Answer from the drawing. Dimensions are ordinates in mm from the lowest x, y and z of the part. A direction names the side the tool comes from. Coordinates: 2 decimals unless noted, no trailing zeros. Order: outer loops, then holes, each group sorted by start corner. A loop starts at its lowest first (then second) coordinate and runs counter-clockwise, first axis right, second up. Notation, with made-up numbers: M 42.5,7.25 L 48.5,7.25 A22 cw 48.5,24.25 Z; hole C 53.5,17.25 d7. An arc over 180 degrees is marked long. One line per question, with ' | ' between items. Start each with the question number.
1) Find section A-A, the plane z = 3. Write down the section's boundary in (x, y).
2) Find section B-B, the plane y = 3. Write down the section's boundary in (x, z).
3) Given P1, Ø0.9, axis at x = 4, z = 3, coming from the +Y side; P2, Ø1, axis at y = 3, z = 5, coming from the +X side; P3, Ø2, axis at x = 1.5, y = 21.5, coming from the +Z side, each flat-ended and moving along its own axis, determine where each tip first touches the part or whether it passes through.
4) Consider probe 1 along Y at (x, z) = (4.95, 3); probe 2 along Z at (x, y) = (4, 15.75); probe 3 along Z at (x, y) = (2.9, 16). Determine where each line is inside the solid, lowest interval first.
5) A tool of negligible diameter and unlimited length cuts with its end or side. For the marked faces 1 and 2, from which of +Z, -Z, +X, -X, +Y, -Y can it reach the whole face along a straight path? Write none if from no direction.
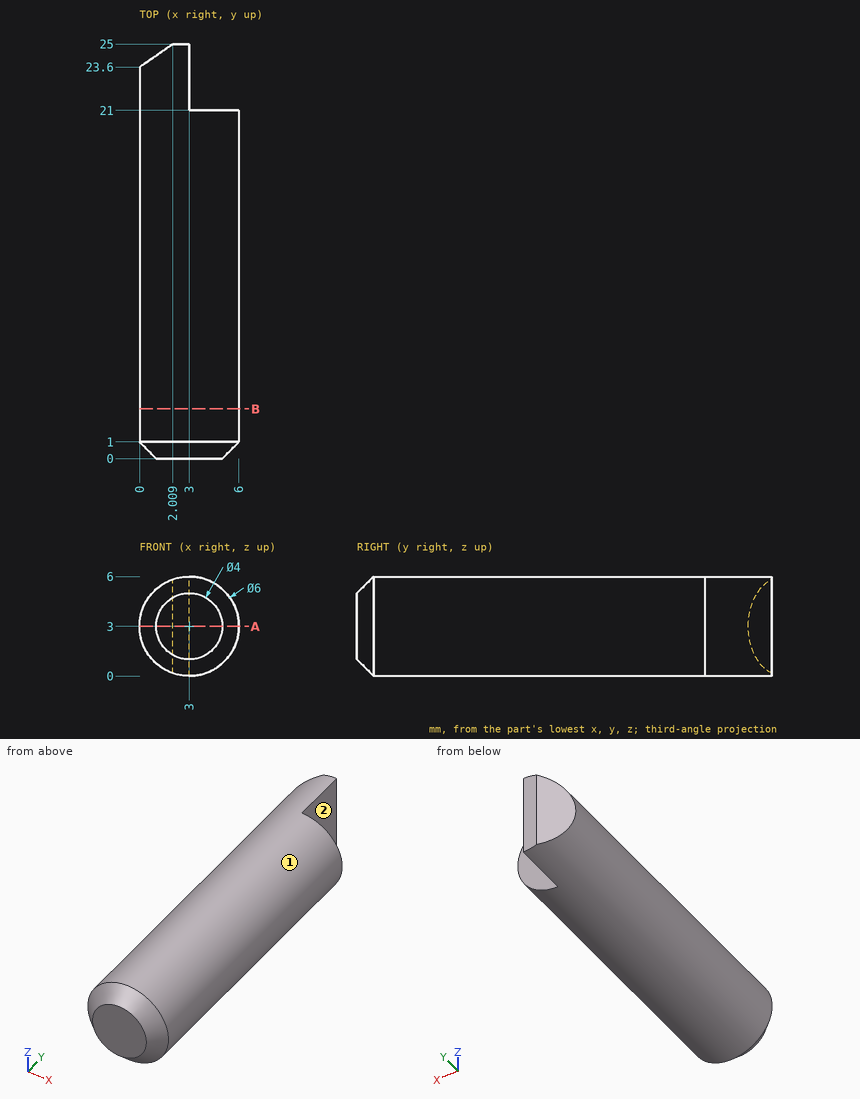
Report:
1) outline: M 0,1 L 1,0 L 5,0 L 6,1 L 6,21 L 3,21 L 3,25 L 2.01,25 L 0,23.6 Z
2) outline: C 3,3 d6
3) P1: stops at y = 21 | P2: stops at x = 5.6 | P3: stops at z = 5.96
4) probe 1: y = 0 to 21 | probe 2: z = 0.17 to 5.83 | probe 3: z = 0 to 6
5) face 1: +Y, -Y | face 2: +Z, -Z, +X, +Y
